from build123d import *

# Parameters (mm, degrees)
ESQUISSE1_R             = 7.5
BOSS_EXTRU_1_DEPTH      = 5
ESQUISSE2_R             = 6
BOSS_EXTRU_2_DEPTH      = 7
ESQUISSE3_R             = 7.5
BOSS_EXTRU_3_DEPTH      = 3
ESQUISSE4_R             = 2.5
ENL_V_MAT_EXTRU_1_DEPTH = 30


with BuildPart() as part:
    # Esquisse1 → Boss.-Extru.1 (new body)
    with BuildSketch(Plane.XY):
        Circle(ESQUISSE1_R)
    extrude(amount=BOSS_EXTRU_1_DEPTH)

    # Esquisse2 → Boss.-Extru.2 (add)
    with BuildSketch(Plane.XY.offset(5)):
        Circle(ESQUISSE2_R)
    extrude(amount=BOSS_EXTRU_2_DEPTH)

    # Esquisse3 → Boss.-Extru.3 (add)
    with BuildSketch(Plane.XY.offset(12)):
        Circle(ESQUISSE3_R)
    extrude(amount=BOSS_EXTRU_3_DEPTH)

    # Esquisse4 → Enlèv. mat.-Extru.1 (cut)
    with BuildSketch(Plane(origin=(0, 0, 0), x_dir=(-1, 0, 0), z_dir=(0, 0, -1))):
        Circle(ESQUISSE4_R)
    extrude(amount=-ENL_V_MAT_EXTRU_1_DEPTH, mode=Mode.SUBTRACT)


solid = part.part
Could you check a few things on this model? Use its own coordinates, in mm. A direction names the side the tool comes from. Round coordinates to 2 decimals unless told otherwise and drop trailing zeros. Write each loop counter-clockwise with the first axis right and the second up, starting at its lowest first coordinate (ties: lowest second). Pieces come first, ordered by that corner, then holes. Notation, with made-up numbers: (22, -29) - (80, -29) arc R13 cw to (80, -16) - close; hole circle Ø8 at (-21, 71.25). An arc over 180 degrees is marked (long way). Use a Markdown table: item, result.
Q1. Thinking about a two-plate mould opening in X: for faces 3 (the cylindrical face through (0.54, -2.44, 7.4)), 4 (the flat face through (2, 6, 12)), 5 (the cylindrical face through (-6, 0, 8)), which applies, released by +X, released by -X, zero draft, split by the parting line, or undercut?
Output values:
| item | result |
|---|---|
| face 3 | undercut |
| face 4 | zero draft |
| face 5 | split by the parting line |
Q2. I want a section at A-A (x = 0). List the corners of the cut face in (y, z) for me.
Output values:
| item | result |
|---|---|
| outline | (-7.5, 0) - (-2.5, 0) - (-2.5, 15) - (-7.5, 15) - (-7.5, 12) - (-6, 12) - (-6, 5) - (-7.5, 5) - close; (2.5, 0) - (7.5, 0) - (7.5, 5) - (6, 5) - (6, 12) - (7.5, 12) - (7.5, 15) - (2.5, 15) - close |
Q3. I want a section at C-C (z = 6.5). List the corners of the cut face in (x, y) for me, plus the area to 3 significant figures.
Output values:
| item | result |
|---|---|
| outline | circle Ø12 at (0, 0); hole circle Ø5 at (0, 0) |
| area | 93.5 mm2 |
Q4. For pin 1 (4 mm diameter, centred on x = 0, y = 0, fed in from -Z); pin 2 (8 mm diameter, centred on x = 5, z = 8, fed in from -Y); pin 3 (6 mm diameter, centred on y = 5.5, z = 3, fed in from -X), each with a flat end and sliding along its axis, tell me the tip position at first contact or that it passes through.
Output values:
| item | result |
|---|---|
| pin 1 | through |
| pin 2 | y = -7.12 |
| pin 3 | x = -7.07 |
Q5. Please list where these lines run through material, in increasing order: L1, parallel to Y at x = 0, z = 10.5; L2, parallel to Z at x = -5.25, y = 3; L3, parallel to Y at x = -0.5, z = 11.5.
Output values:
| item | result |
|---|---|
| L1 | -6 to -2.5, 2.5 to 6 |
| L2 | 0 to 5, 12 to 15 |
| L3 | -5.98 to -2.45, 2.45 to 5.98 |
Q6. For faces 1 (the flat face through (-2, 2, 0)), 2 (the flat face through (2, 6, 5)), which set-ups out of +Z, -Z, +X, -X, +Y, -Y let a thin tool reach every point of the face, with its end or its side?
Output values:
| item | result |
|---|---|
| face 1 | -Z, +X, -X, +Y, -Y |
| face 2 | none |
Q7. I want a section at D-D (x = -2.75). List the corners of the cut face in (y, z) for me.
Output values:
| item | result |
|---|---|
| outline | (-6.98, 0) - (6.98, 0) - (6.98, 5) - (5.33, 5) - (5.33, 12) - (6.98, 12) - (6.98, 15) - (-6.98, 15) - (-6.98, 12) - (-5.33, 12) - (-5.33, 5) - (-6.98, 5) - close |
